from build123d import *

# Parameters (mm, degrees)
SKETCH1_R           = 6.3627
BOSS_EXTRUDE1_DEPTH = 3.175


with BuildPart() as part:
    # Sketch1 → Boss-Extrude1 (new body, symmetric)
    with BuildSketch(Plane.XY):
        with BuildLine():
            ThreePointArc((-15.719319348, -43.426177466), (-9.406121761, -57.631125381), (-7.246114065, -73.025))
            Line((-7.246114065, -73.025), (19.05, -73.025))
            Line((19.05, -73.025), (19.05, 73.025))
            Line((19.05, 73.025), (-7.246114065, 73.025))
            ThreePointArc((-7.246114065, 73.025), (-9.406121761, 57.631125381), (-15.719319348, 43.426177466))
            ThreePointArc((-15.719319348, 43.426177466), (1.415517775, 24.650338319), (7.62, 0))
            ThreePointArc((7.62, 0), (1.415517775, -24.650338319), (-15.719319348, -43.426177466))
        make_face()
        with Locations((6.35, -60.325)):
            Circle(SKETCH1_R, mode=Mode.SUBTRACT)
        with Locations((6.35, 60.325)):
            Circle(SKETCH1_R, mode=Mode.SUBTRACT)
    extrude(amount=BOSS_EXTRUDE1_DEPTH, both=True)


solid = part.part
Geometry: final body of the model. Coordinates: model frame, mm. Give positions to 0.01 mm unless a question says otherwise; leave off trailing zeros. Order: outer loops, then holes, each group sorted by start corner. A loop starts at its lowest first (then second) coordinate and runs counter-clockwise, first axis right, second up. Notation, with made-up numbers: (26.25, -38) -> (34.25, -38) arc R28 ccw to (34.25, -2) -> close; hole circle Ø8 at (79, 0.25). An arc over 180 degrees is marked (long way). Answer as a JSON object with one key per item and string values.
Q1. Section D-D (x = -11). Output: boundary loops of the cut face in (y, z) (3 decimals), plus the area to 3 significant figures.
Entries:
{"outline": "(-52.879, -3.175) -> (-39.905, -3.175) -> (-39.905, 3.175) -> (-52.879, 3.175) -> close; (39.905, -3.175) -> (52.879, -3.175) -> (52.879, 3.175) -> (39.905, 3.175) -> close", "area": "165 mm^2"}
Q2. Material intervals for probe 1 along Y at (x, z) = (-1, -2.25) (3 decimals); probe 2 along X at (y, z) = (60, -2.75); probe 3 along X at (y, z) = (-65, -1.75), sorted ascending.
Entries:
{"probe 1": "y = -73.025 to -28.695, 28.695 to 73.025", "probe 2": "x = -8.78 to 0, 12.7 to 19.05", "probe 3": "x = -7.82 to 2.03, 10.67 to 19.05"}
Q3. First-contact query: pin 1 (16.5 mm diameter, centred on x = 6.35, y = -60.325, fed in from -Z) (3 decimals); pin 2 (1.5 mm diameter, centred on y = -21, z = 0.5, fed in from -X). Flat tips, straight axial feed; report the tip coordinate or a pass-through.
Entries:
{"pin 1": "stops at z = -3.175", "pin 2": "stops at x = 2.86"}
Q4. Section C-C (z = -1.5). Output: boundary loops of the cut face in (x, y) (3 decimals).
Entries:
{"outline": "(-15.719, -43.426) arc R55.934 cw to (-7.246, -73.025) -> (19.05, -73.025) -> (19.05, 73.025) -> (-7.246, 73.025) arc R55.934 cw to (-15.719, 43.426) arc R52.07 cw to start; hole circle Ø12.725 at (6.35, -60.325); hole circle Ø12.725 at (6.35, 60.325)"}
Q5. Draft query along Y for faces 1 (the flat face through (9, 1, 3.175)), 2 (the cylindrical face through (-9.467, -57.421, 0.044)), 3 (the cylindrical face through (7.615, 0.719, 0.044)). Return one class per face: released by +Y, released by -Y, zero draft, split by the parting line, or undercut.
Entries:
{"face 1": "zero draft", "face 2": "released by -Y", "face 3": "undercut"}
Q6. Section B-B (x = -5). Output: boundary loops of the cut face in (y, z) (3 decimals).
Entries:
{"outline": "(-73.025, -3.175) -> (-33.985, -3.175) -> (-33.985, 3.175) -> (-73.025, 3.175) -> close; (33.985, -3.175) -> (73.025, -3.175) -> (73.025, 3.175) -> (33.985, 3.175) -> close"}
Q7. Section A-A (x = 6.35). Output: boundary loops of the cut face in (y, z) (3 decimals).
Entries:
{"outline": "(-73.025, -3.175) -> (-66.688, -3.175) -> (-66.688, 3.175) -> (-73.025, 3.175) -> close; (-53.962, -3.175) -> (-11.43, -3.175) -> (-11.43, 3.175) -> (-53.962, 3.175) -> close; (11.43, -3.175) -> (53.962, -3.175) -> (53.962, 3.175) -> (11.43, 3.175) -> close; (66.688, -3.175) -> (73.025, -3.175) -> (73.025, 3.175) -> (66.688, 3.175) -> close"}
